```python
from build123d import *

# Parameters (mm, degrees)
F0_R            = 11
F1_DEPTH        = 8
F2_DEPTH        = 8
F2_COPIES_COUNT = 3
F3_R            = 5.08
F4_F1_R         = 0.762
F4_F2_R         = 0.762
F4_F3_R         = 0.762
F5_SIZE         = 0.762


# Not quite as in the source:
# - a pattern or mirror of a feature is missing from the dataset's text; its kind, count and spacing are read off the source's solid


with BuildPart() as f1:
    # F0 (on Top) → F1 (new body)
    with BuildSketch(Plane.XY):
        with BuildLine():
            ThreePointArc((-11.407337121, 9.7402597403), (-5.190854611, -14.0732024929), (15, 0))
            ThreePointArc((15, 0), (10.6066017178, 10.6066017178), (0, 15))
            ThreePointArc((0, 15), (-6.2807684202, 13.6217454114), (-11.407337121, 9.7402597403))
        make_face()
        Circle(F0_R, mode=Mode.SUBTRACT)
    extrude(amount=-F1_DEPTH)

    # F0 (on Top) → F2 (join, through all)
    with BuildSketch(Plane.XY):
        with BuildLine():
            ThreePointArc((-11.407337121, 9.7402597403), (-6.2807684202, 13.6217454114), (0, 15))
            Line((0, 15), (11.407337121, 28.3597402597))
            ThreePointArc((11.407337121, 28.3597402597), (6.2807684202, 24.4782545886), (0, 23.1))
            Line((0, 23.1), (-11.407337121, 9.7402597403))
        make_face()
        with BuildLine():
            ThreePointArc((0, 23.1), (6.2807684202, 24.4782545886), (11.407337121, 28.3597402597))
            ThreePointArc((11.407337121, 28.3597402597), (14.0732024929, 32.909145389), (15, 38.1))
            ThreePointArc((15, 38.1), (10.6066017178, 48.7066017178), (0, 53.1))
            ThreePointArc((0, 53.1), (-4.9701878524, 52.2526404855), (-9.378837576, 49.806297695))
            ThreePointArc((-9.378837576, 49.806297695), (-14.1526404855, 33.1298121476), (0, 23.1))
        make_face()
        with Locations((0, 38.1)):
            Circle(F0_R, mode=Mode.SUBTRACT)
        with BuildLine():
            Line((11.407337121, 66.4597402597), (-9.378837576, 49.806297695))
            ThreePointArc((-9.378837576, 49.806297695), (-4.9701878524, 52.2526404855), (0, 53.1))
            Line((0, 53.1), (11.407337121, 66.4597402597))
        make_face()
    f2 = extrude(amount=-F2_DEPTH)

    # F2_copies: F2 ×3 about axis
    f2_copies_axis = Axis((0, 0, 0), (0, 0, 1))
    for i in range(1, F2_COPIES_COUNT):
        add(f2.rotate(f2_copies_axis, i * 360 / F2_COPIES_COUNT))

    # F3
    f3_edges = [f1.edges().sort_by_distance(p)[0] for p in [
        (0, 15, -4),
        (0, 23.1, -4),
        (0, 53.1, -4),
        (20.005187, -11.55, -4),
        (-12.990381, -7.5, -4),
        (-45.985949, -26.55, -4),
        (-20.005187, -11.55, -4),
        (12.990381, -7.5, -4),
        (45.985949, -26.55, -4),
    ]]
    fillet(f3_edges, radius=F3_R)

    # F4: fillet of radius 0.762 on 3 edges, made by hand

    # F4_f1
    f4_f1_edges = [f1.edges().sort_by_distance(p)[0] for p in [
        (51.8521548333, -43.1089138662, -4),
    ]]
    fillet(f4_f1_edges, radius=F4_F1_R)

    # F4_f2
    f4_f2_edges = [f1.edges().sort_by_distance(p)[0] for p in [
        (11.407337121, 66.4597402597, -4),
    ]]
    fillet(f4_f2_edges, radius=F4_F2_R)

    # F4_f3
    f4_f3_edges = [f1.edges().sort_by_distance(p)[0] for p in [
        (-63.2594919544, -23.3508263935, -4),
    ]]
    fillet(f4_f3_edges, radius=F4_F3_R)

    # F5
    f5_edges = [f1.edges().sort_by_distance(p)[0] for p in [
        (-11, 0, 0),
        (-11, 38.1, 0),
        (-11, 38.1, -8),
        (-27.495568, -28.576279, -8),
        (38.495568, -9.523721, -8),
        (-27.495568, -28.576279, 0),
        (38.495568, -9.523721, 0),
    ]]
    chamfer(f5_edges, length=F5_SIZE)


solid = f1.part
```
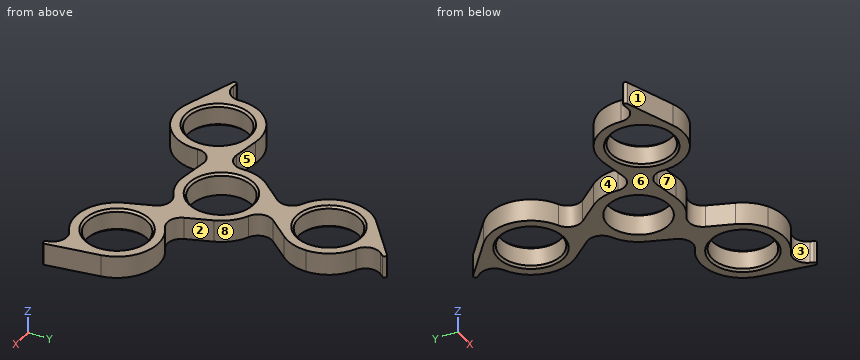
Design review of the part built by this model. Coordinates are the model's own, in mm. Face numbers are marked on the shaded views. A direction names the side the tool comes from. Coordinates: 2 decimals unless noted, no trailing zeros. Order: outer loops, then holes, each group sorted by start corner. A loop starts at its lowest first (then second) coordinate and runs counter-clockwise, first axis right, second up. Notation, with made-up numbers: (33.25, 38.25) - (67.25, 38.25) arc R12 ccw to (67.25, 55.25) - close; hole circle Ø2 at (61, 46). An arc over 180 degrees is marked (long way). One line per question, with ' | ' between items.
Q1. The part is to be moulded in two halves that separate along X. For the marked faces 1, 2 and 3, say which applies: +X half, -X half, draft (parallel to the pull), parting line (faces both ways), or undercut.
Answer key:
face 1: -X half | face 2: +X half | face 3: undercut
Q2. Clearance check with flat-ended pins moving along their axes: pin 1 Ø2 at (y, z) = (-7, -7) entering from -X; pin 2 Ø3 at (x, z) = (-4, -5) entering from -Y; pin 3 Ø20 at (x, y) = (-33, -19.05) entering from -Z; pin 4 Ø3 at (y, z) = (29.5, -4.5) entering from -X. State where each tip first meets the part, or that it passes through.
Answer key:
pin 1: stops at x = -43.14 | pin 2: stops at y = -14.79 | pin 3: passes through | pin 4: stops at x = -13.21
Q3. Consider section B-B, the plane z = -3. Give the number of separate pieces and of enclosed holes in the cut face, then the cut area to 3 significant figures.
Answer key:
separate pieces: 1 | enclosed holes: 4 | area: 1,730 mm2
Q4. To check wall thickness, follow line 1 along Y through (x, z) = (-4.5, -5.25); line 2 along X through (y, z) = (37.5, -3); line 3 along Y through (x, z) = (0, -5). State the ranges of each line that lie inside material, in increasing order.
Answer key:
line 1: y = -14.42 to -10.04, 10.04 to 18.15, 22.29 to 28.06, 48.14 to 53.72 | line 2: x = -14.99 to -10.98, 10.98 to 14.99 | line 3: y = -15 to -11, 11 to 27.1, 49.1 to 57.32
Q5. For the marked faces 4, 5, 6, 7 and 8, list the 3-axis set-ups (+Z, -Z, +X, -X, +Y, -Y) from which the entire face can be reached by the end or side of a thin tool; tool diameter is ignored.
Answer key:
face 4: +Z, -Z, -X | face 5: +Z, -Z, +Y | face 6: -Z, +X, -X, +Y, -Y | face 7: +Z, -Z, -Y | face 8: +Z, -Z, +X
Q6. Consider section A-A, the plane x = 0. Give the boundary of the cut face in (y, z), then the cut area to 3 significant figures.
Answer key:
outline: (-15, -8) - (-11, -8) - (-11, -0.76) - (-11.76, 0) - (-15, 0) - close; (11, -8) - (26.34, -8) - (27.1, -7.24) - (27.1, -0.76) - (26.34, 0) - (11.76, 0) - (11, -0.76) - close; (49.1, -7.24) - (49.86, -8) - (57.32, -8) - (57.32, 0) - (49.86, 0) - (49.1, -0.76) - close | area: 225 mm2
